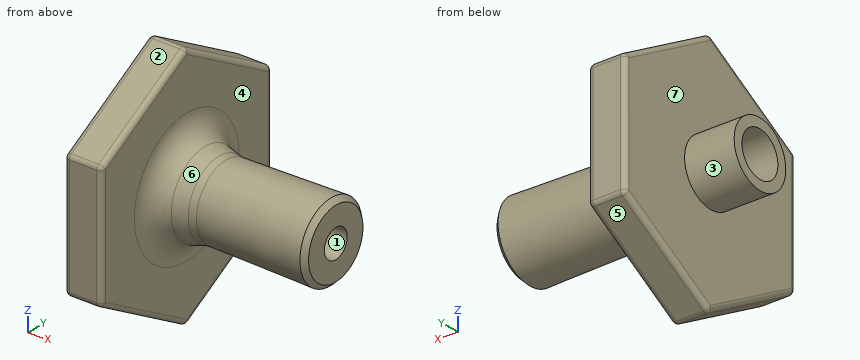
from build123d import *

# Parameters (mm, degrees)
FILLET4_R               = 3
CHAMFER1_SIZE2          = 0.393197641
CHAMFER1_SIZE           = 0.4
CUT_EXTRUDE1_DEPTH      = 13.023098533
CUT_EXTRUDE1_DEPTH_BACK = 8.0000001
FILLET5_R               = 0.4
FILLET6_R               = 2


with BuildPart() as part:
    # Sketch1 → Revolve1 (revolve)
    with BuildSketch(Plane.XY):
        Polygon((0, 1.825), (6.718918331, 1.825), (9.596035247, 1), (19.023098433, 1.16455), (19.023098433, 3.164854656), (9.859986912, 3.00491195), (7, 3.825), (7, 10), (4, 10), (4, 2.625), (0, 2.625), align=None)
    revolve(axis=Axis((0, 0, 0), (1, 0, 0)))

    # Fillet4
    fillet4_edges = [part.edges().sort_by_distance(p)[0] for p in [
        (9.596035247, -1, 0),
        (6.718918331, -1.825, 0),
    ]]
    fillet(fillet4_edges, radius=FILLET4_R)

    # Chamfer1
    chamfer1_edges = [part.edges().sort_by_distance(p)[0] for p in [
        (19.023098433, -3.164854656, 0),
    ]]
    chamfer(chamfer1_edges, length=CHAMFER1_SIZE, length2=CHAMFER1_SIZE2)

    # Sketch2 → Cut-Extrude1 (cut, two sides)
    with BuildSketch(Plane(origin=(7, 0, 0), x_dir=(0, 0, -1), z_dir=(1, 0, 0))) as cut_extrude1_sk:
        with BuildLine():
            Line((-10, 0), (-5, 8.660254038))
            ThreePointArc((-5, 8.660254038), (-8.660254038, 5), (-10, 0))
        make_face()
        with BuildLine():
            Line((-5, 8.660254038), (5, 8.660254038))
            ThreePointArc((5, 8.660254038), (0, 10), (-5, 8.660254038))
        make_face()
        with BuildLine():
            Line((5, 8.660254038), (10, 0))
            ThreePointArc((10, 0), (8.660254038, 5), (5, 8.660254038))
        make_face()
        with BuildLine():
            ThreePointArc((-10, 0), (-8.660254038, -5), (-5, -8.660254038))
            Line((-5, -8.660254038), (-10, 0))
        make_face()
        with BuildLine():
            ThreePointArc((-5, -8.660254038), (0, -10), (5, -8.660254038))
            Line((5, -8.660254038), (-5, -8.660254038))
        make_face()
        with BuildLine():
            ThreePointArc((5, -8.660254038), (8.660254038, -5), (10, 0))
            Line((10, 0), (5, -8.660254038))
        make_face()
    extrude(amount=CUT_EXTRUDE1_DEPTH, mode=Mode.SUBTRACT)
    extrude(cut_extrude1_sk.sketch, amount=-CUT_EXTRUDE1_DEPTH_BACK, mode=Mode.SUBTRACT)

    # Fillet5
    fillet5_edges = [part.edges().sort_by_distance(p)[0] for p in [
        (7, -4.330127019, -7.5),
        (4, -4.330127019, -7.5),
        (4, -8.660254038, 0),
        (4, 4.330127019, -7.5),
        (4, 4.330127019, 7.5),
        (5.5, 8.660254038, 5),
        (7, 4.330127019, 7.5),
        (5.5, 0, 10),
        (5.5, 0, -10),
        (7, 4.330127019, -7.5),
        (5.5, 8.660254038, -5),
        (5.5, -8.660254038, 5),
        (7, -8.660254038, 0),
        (5.5, -8.660254038, -5),
        (7, 8.660254038, 0),
        (4, 8.660254038, 0),
        (7, -4.330127019, 7.5),
        (4, -4.330127019, 7.5),
    ]]
    fillet(fillet5_edges, radius=FILLET5_R)

    # Fillet6
    fillet6_edges = [part.edges().sort_by_distance(p)[0] for p in [
        (7, -3.825, 0),
        (9.859986912, -3.00491195, 0),
    ]]
    fillet(fillet6_edges, radius=FILLET6_R)


solid = part.part
The model under review builds one solid part; all positions refer to its coordinate system, in mm. Face numbers are marked on the shaded views. A direction names the side the tool comes from. Round coordinates to 2 decimals unless told otherwise and drop trailing zeros. Order: outer loops, then holes, each group sorted by start corner. A loop starts at its lowest first (then second) coordinate and runs counter-clockwise, first axis right, second up. Notation, with made-up numbers: (30.25, -22.75) -> (57.25, -22.75) arc R13 cw to (57.25, -17.75) -> close; hole circle Ø11 at (-10.5, 51.25). An arc over 180 degrees is marked (long way). Write item = value, one per line. Start each with the question number.
Item 1: For line 1 along Z through (x, y) = (3, 0) (3 decimals); line 2 along Y through (x, z) = (4.75, 0) (3 decimals); line 3 along Z through (x, y) = (5.25, 0) (3 decimals), list the stretches that pass through material, from the lowest coordinate up.
Item 2: Consider section A-A on x = 12.75. Write out the cut boundary in (y, z).
Item 3: Mouldability with a two-part tool opening along Y and no side actions: class the marked faces 1, 2 and 3 as released by +Y, released by -Y, zero draft, split by the parting line, or undercut.
Item 4: Clearance check with flat-ended pins moving along their axes: pin 1 Ø8 at (x, y) = (6, -5) entering from +Z; pin 2 Ø3 at (x, y) = (7.5, -3.5) entering from +Z; pin 3 Ø5 at (x, y) = (10, -2.5) entering from -Z. State where each tip first meets the part, or that it passes through.
Item 5: For the marked faces 4, 5, 6 and 7, list the 3-axis set-ups (+Z, -Z, +X, -X, +Y, -Y) from which the entire face can be reached by the end or side of a thin tool; tool diameter is ignored.
Conclusion:
q1.line_1 = -2.625 to -1.825, 1.825 to 2.625
q1.line_2 = -8.66 to -1.825, 1.825 to 8.66
q1.line_3 = -9.938 to -1.825, 1.825 to 9.938
q2.outline = circle Ø6.11 at (0, 0); hole circle Ø2.11 at (0, 0)
q3.face_1 = undercut
q3.face_2 = released by -Y
q3.face_3 = split by the parting line
q4.pin_1 = 9.42
q4.pin_2 = 8.7
q4.pin_3 = -3.5
q5.face_4 = +X
q5.face_5 = -Z, +X, -X, +Y
q5.face_6 = none
q5.face_7 = -X
